Read the model definition and answer for the solid it produces. Units are mm, in the model's axes. Face numbers are marked on the shaded views. A direction names the side the tool comes from. Give positions to 0.01 mm unless a question says otherwise; leave off trailing zeros. Order: outer loops, then holes, each group sorted by start corner. A loop starts at its lowest first (then second) coordinate and runs counter-clockwise, first axis right, second up. Notation, with made-up numbers: M -1.5,30 L 35.5,30 A21 cw 35.5,44 Z; hole C 86.25,81 d7. An arc over 180 degrees is marked long. Write item = value, one per line. Start each with the question number.
from build123d import *

# Parameters (mm, degrees)
SKETCH1_R           = 3.75
BOSS_EXTRUDE1_DEPTH = 7
SKETCH3_R           = 3.75
SKETCH3_R_2         = 3.25
CUT_EXTRUDE1_DEPTH  = 2
SKETCH4_R           = 1.75
CUT_EXTRUDE2_DEPTH  = 6.5
SKETCH5_R           = 2.5
CUT_EXTRUDE4_DEPTH  = 1


with BuildPart() as part:
    # Sketch1 → Boss-Extrude1 (new body)
    with BuildSketch(Plane(origin=(0, 0, 0), x_dir=(1, 0, 0), z_dir=(0, 1, 0))):
        Circle(SKETCH1_R)
    extrude(amount=BOSS_EXTRUDE1_DEPTH)

    # Sketch3 → Cut-Extrude1 (cut)
    with BuildSketch(Plane(origin=(0, 7, 0), x_dir=(1, 0, 0), z_dir=(0, 1, 0))):
        Circle(SKETCH3_R)
        Circle(SKETCH3_R_2, mode=Mode.SUBTRACT)
    extrude(amount=-CUT_EXTRUDE1_DEPTH, mode=Mode.SUBTRACT)

    # Sketch4 → Cut-Extrude2 (cut)
    with BuildSketch(Plane(origin=(0, 7, 0), x_dir=(1, 0, 0), z_dir=(0, 1, 0))):
        Circle(SKETCH4_R)
    extrude(amount=-CUT_EXTRUDE2_DEPTH, mode=Mode.SUBTRACT)

    # Sketch5 → Cut-Extrude4 (cut)
    with BuildSketch(Plane(origin=(0, 7, 0), x_dir=(1, 0, 0), z_dir=(0, 1, 0))):
        Circle(SKETCH5_R)
    extrude(amount=-CUT_EXTRUDE4_DEPTH, mode=Mode.SUBTRACT)


solid = part.part
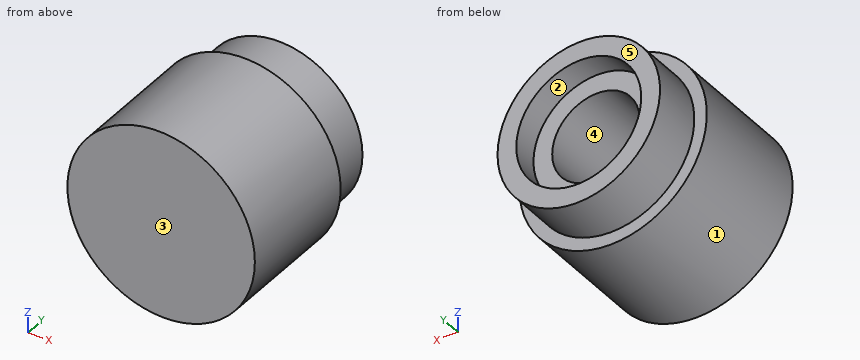
1) For a pull along Z with two mould halves and no side action, classify the marked faces 1, 2 and 3 as pulls with the +Z half, pulls with the -Z half, needs draft (parallel to the pull), parting line crosses it, or undercut.
2) Find section A-A on x = 0. Determine the outline of the cut face in (y, z).
3) For the marked faces 4 and 5, determine the directions among +Z, -Z, +X, -X, +Y, -Y from which every point of the face is accessible in a straight line to the end or side of a thin tool.
4) Find section D-D on x = -2.75. Determine the outline of the cut face in (y, z).
5) Find the intervals of material crossed by probe 1 along Z at (x, y) = (0, 3.1); probe 2 along Y at (x, z) = (1, -1), in increasing order. Write a range as [from, to].
6) Each of these flat-tipped pins is pushed along its axis until it touches: P1, Ø2, axis at x = 0, z = 0, coming from the -Y side; P2, Ø3, axis at x = -0.5, z = -0.5, coming from the +Y side; P3, Ø1.5, axis at y = 5, z = 1.5, coming from the +X side; P4, Ø3, axis at y = 3, z = 2.5, coming from the +X side. Where does it stop, or does it pass through?
7) Find section B-B on z = 0. Determine the outline of the cut face in (x, y).
8) Find section C-C on y = 6.5. Determine the outline of the cut face in (x, z).
Numbers:
q1.face_1 = parting line crosses it
q1.face_2 = undercut
q1.face_3 = needs draft
q2.outline = M 0,-3.75 L 5,-3.75 L 5,-3.25 L 7,-3.25 L 7,-2.5 L 6,-2.5 L 6,-1.75 L 0.5,-1.75 L 0.5,1.75 L 6,1.75 L 6,2.5 L 7,2.5 L 7,3.25 L 5,3.25 L 5,3.75 L 0,3.75 Z
q3.face_4 = +Y
q3.face_5 = +Z, -Z, +X, -X, +Y
q4.outline = M 0,-2.55 L 5,-2.55 L 5,-1.73 L 7,-1.73 L 7,1.73 L 5,1.73 L 5,2.55 L 0,2.55 Z
q5.probe_1 = [-3.75, -1.75], [1.75, 3.75]
q5.probe_2 = [0, 0.5]
q6.P1 = 0
q6.P2 = 6
q6.P3 = 3.67
q6.P4 = 3.61
q7.outline = M -3.75,0 L 3.75,0 L 3.75,5 L 3.25,5 L 3.25,7 L 2.5,7 L 2.5,6 L 1.75,6 L 1.75,0.5 L -1.75,0.5 L -1.75,6 L -2.5,6 L -2.5,7 L -3.25,7 L -3.25,5 L -3.75,5 Z
q8.outline = C 0,0 d6.5; hole C 0,0 d5
